from build123d import *

# Parameters (mm, degrees)
F1_DEPTH = 3.175
F3_DEPTH = 9.525
F5_DEPTH = 3.176


# Not quite as in the source:
# - a feature names something its author has since deleted; it is built from what else it names


with BuildPart() as f1:
    # F0 (on Front) → F1 (new body)
    with BuildSketch(Plane.XZ):
        with BuildLine():
            Line((101.6, 6.35), (-101.6, 6.35))
            Line((-101.6, 6.35), (-101.6, -6.35))
            Line((-101.6, -6.35), (-92.5598257878, -40.0883894691))
            Line((-92.5598257878, -40.0883894691), (-92.075, -40.6661823435))
            Line((-92.075, -40.6661823435), (-92.075, -34.925))
            Line((-92.075, -34.925), (-88.9, -34.925))
            Line((-88.9, -34.925), (-88.9, -15.875))
            ThreePointArc((-88.9, -15.875), (-89.4567758795, -15.6443758795), (-89.6874, -15.0876))
            Line((-89.6874, -15.0876), (-89.6874, -6.35))
            Line((-89.6874, -6.35), (101.6, -6.35))
            Line((101.6, -6.35), (101.6, 6.35))
        make_face()
    extrude(amount=F1_DEPTH)

    # F2 (on face) → F3 (join)
    with BuildSketch(Plane(origin=(0, 0, -34.925), x_dir=(1, 0, 0), z_dir=(0, 0, -1))):
        Polygon((-88.9, 0), (-92.075, 3.175), (-92.075, 0), align=None)
    extrude(amount=F3_DEPTH)

    # F4 (on face) → F5 (cut, through all)
    with BuildSketch(Plane(origin=(0, 0, 0), x_dir=(-1, 0, 0), z_dir=(0, 1, 0))):
        Polygon((92.075, -44.45), (92.075, -40.6661823435), (88.9, -44.45), align=None)
    extrude(amount=-F5_DEPTH, mode=Mode.SUBTRACT)


solid = f1.part
Read the model definition and answer for the solid it produces. Units are mm, in the model's axes. A direction names the side the tool comes from. Round coordinates to 2 decimals unless told otherwise and drop trailing zeros. Order: outer loops, then holes, each group sorted by start corner. A loop starts at its lowest first (then second) coordinate and runs counter-clockwise, first axis right, second up. Notation, with made-up numbers: (29.5, 4) - (66.5, 4) arc R29 ccw to (66.5, 36) - close; hole circle Ø5 at (49, -10). An arc over 180 degrees is marked (long way). Use one line per item in the form item = value. Start each with the question number.
(1) Determine the mould class of faces 1 (the face through (-97.143, -1.565, -22.983)), 2 (the face through (1, -2, 6.35)), 3 (the face through (-8, -3.175, -3)), 4 (the face through (-89.687, -2, -11)) for opening direction Z: +Z half, -Z half, draft (parallel to the pull), parting line (faces both ways), or undercut.
(2) The part is cut by section B-B (x = -68). Give the vertices of the cut face in (y, z) (3 decimals), then the cut area to 3 significant figures.
(3) The part is cut by section C-C (z = -19). Give the vertices of the cut face in (x, y) (3 decimals), then the cut area to 3 significant figures.
(4) The part is cut by section A-A (y = -2.1). Give the vertices of the cut face in (x, z) (3 decimals), then the cut area to 3 significant figures.
(5) Flat-ended cylindrical pins translate along their axes: pin 1 Ø1.6 at (x, y) = (36, -1) entering from -Z; pin 2 Ø1 at (x, y) = (-90, -2.5) entering from -Z (3 decimals); pin 3 Ø3 at (x, z) = (-12.5, -9.5) entering from -Y. Find the tip coordinate at first contact, or state that the pin passes through.
(6) Find the intervals of material crossed by line 1 along Z through (x, y) = (21, -2.65); line 2 along X through (y, z) = (-0.95, -13); line 3 along X through (y, z) = (-1.65, -16.5), in increasing order. Write a range as from..to.
(7) For faces 5 (the face through (101.6, -2, 0)), 6 (the face through (-90.5, -1.6, -38.6)), 7 (the face through (-88.9, -2, -26)), determine the directions among +Z, -Z, +X, -X, +Y, -Y from which every point of the face is accessible in a straight line to the end or side of a thin tool.
Checked values:
q1.face_1 = -Z half
q1.face_2 = +Z half
q1.face_3 = draft
q1.face_4 = undercut
q2.outline = (-3.175, -6.35) - (0, -6.35) - (0, 6.35) - (-3.175, 6.35) - close
q2.area = 40.3 mm^2
q3.outline = (-98.21, -3.175) - (-88.9, -3.175) - (-88.9, 0) - (-98.21, 0) - close
q3.area = 29.6 mm^2
q4.outline = (-101.6, -6.35) - (-92.56, -40.088) - (-91, -41.947) - (-91, -34.925) - (-88.9, -34.925) - (-88.9, -15.875) arc R0.787 cw to (-89.687, -15.088) - (-89.687, -6.35) - (101.6, -6.35) - (101.6, 6.35) - (-101.6, 6.35) - close
q4.area = 2,840 mm^2
q5.pin_1 = -6.35
q5.pin_2 = -34.925
q5.pin_3 = through
q6.line_1 = -6.35..6.35
q6.line_2 = -99.82..-89.69
q6.line_3 = -98.88..-88.9
q7.face_5 = +Z, -Z, +X, +Y, -Y
q7.face_6 = -Z, +X, -Y
q7.face_7 = -Z, +X, +Y, -Y
